The model under review builds one solid part; all positions refer to its coordinate system, in mm. Give positions to 0.01 mm unless a question says otherwise; leave off trailing zeros. Write each loop counter-clockwise with the first axis right and the second up, starting at its lowest first coordinate (ties: lowest second). Pieces come first, ordered by that corner, then holes. Notation, with made-up numbers: (70, 7) - (106, 7) arc R21 cw to (106, 38) - close; hole circle Ø6 at (38.25, 34.5). An arc over 180 degrees is marked (long way). Write item = value, one per line.
```python
from build123d import *

# Parameters (mm, degrees)
SKETCH_1_W          = 40
SKETCH_1_H          = 20
SKETCH_1_W_2        = 38
SKETCH_1_H_2        = 18
EXTRUDE_1_DEPTH     = 550
SKETCH_4_R          = 1.75
CUT_EXTRUDE_2_DEPTH = 1.5
SKETCH_6_R          = 2.5
CUT_EXTRUDE_3_DEPTH = 552.815186453
SKETCH_7_R          = 1.6
CUT_EXTRUDE_4_DEPTH = 10


with BuildPart() as part:
    # 草图1 → 拉伸-薄壁1 (new body)
    with BuildSketch(Plane.XY):
        with Locations((20, -10)):
            Rectangle(SKETCH_1_W, SKETCH_1_H)
        with Locations((20, -10)):
            Rectangle(SKETCH_1_W_2, SKETCH_1_H_2, mode=Mode.SUBTRACT)
    extrude(amount=EXTRUDE_1_DEPTH)

    # 草图4 → 切除-拉伸2 (cut)
    with BuildSketch(Plane.ZY):
        with Locations((539.996387591, -10)):
            Circle(SKETCH_4_R)
        with Locations((10, -10.000000002)):
            Circle(SKETCH_4_R)
    extrude(amount=-CUT_EXTRUDE_2_DEPTH, mode=Mode.SUBTRACT)

    # 草图6 → 切除-拉伸3 (cut, through all)
    with BuildSketch(Plane(origin=(40, 0, 0), x_dir=(0, 0, -1), z_dir=(1, 0, 0))):
        with Locations((-320, -10)):
            Circle(SKETCH_6_R)
        with Locations((-230, -10)):
            Circle(SKETCH_6_R)
    extrude(amount=-CUT_EXTRUDE_3_DEPTH, mode=Mode.SUBTRACT)

    # 草图7 → 切除-拉伸4 (cut)
    with BuildSketch(Plane.ZY):
        with Locations((190, -10)):
            Circle(SKETCH_7_R)
        with Locations((170, -10)):
            Circle(SKETCH_7_R)
    extrude(amount=-CUT_EXTRUDE_4_DEPTH, mode=Mode.SUBTRACT)


solid = part.part
```
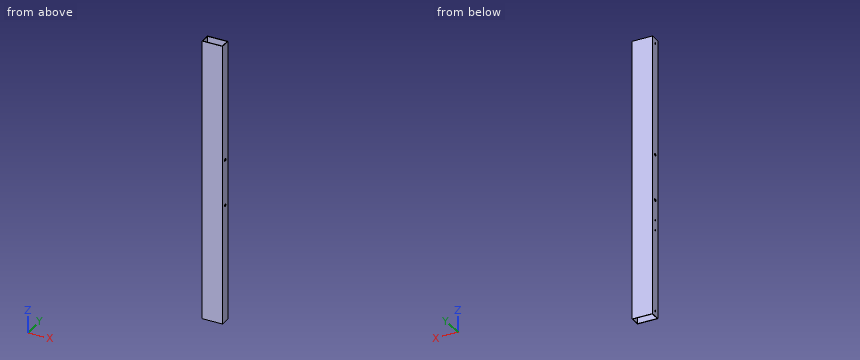
1. For line 1 (Y direction, x = 39.8, z = 320); line 2 (Y direction, x = 7, z = 372); line 3 (X direction, y = -14.25, z = 35.5), list the stretches that pass through material, from the lowest coordinate up. Write a range as from..to.
Findings below:
line_1 = -20..-12.5, -7.5..0
line_2 = -20..-19, -1..0
line_3 = 0..1, 39..40
2. Take a section at A-A on z = 265.5. Give the boundary of the cut face in (x, y).
Findings below:
outline = (0, -20) - (40, -20) - (40, 0) - (0, 0) - close; hole (1, -19) - (39, -19) - (39, -1) - (1, -1) - close
3. Take a section at C-C on x = 18. Give the boundary of the cut face in (y, z), and give its area (3 significant figures).
Findings below:
outline = (-20, 0) - (-19, 0) - (-19, 550) - (-20, 550) - close; (-1, 0) - (0, 0) - (0, 550) - (-1, 550) - close
area = 1,100 mm²
4. Insertion check: P1, Ø3, axis at y = -10, z = 10, coming from the -X side. The pin has a flat end and moves straight along its axis. Give the tip position at first contact, or say it passes through.
Findings below:
P1 = 39
5. Take a section at B-B on y = -4.5. Give the boundary of the cut face in (x, z), and give its area (3 significant figures).
Findings below:
outline = (0, 0) - (1, 0) - (1, 550) - (0, 550) - close; (39, 0) - (40, 0) - (40, 550) - (39, 550) - close
area = 1,100 mm²
